```python
from build123d import *

# Parameters (mm, degrees)
TORUS001_R   = 3.1
BOX_W        = 135
BOX_H        = 90
BOX_DEPTH    = 75
POCKET_DEPTH = 70


with BuildPart() as torus001:
    # Torus001 → Torus001 (revolve)
    with BuildSketch(Plane(origin=(-20, 0, 79), x_dir=(1, 0, 0), z_dir=(0, -1, 0))):
        with Locations((35, 0)):
            Circle(TORUS001_R)
    revolve(axis=Axis((-20, 0, 79), (0, 0, 1)))


with BuildPart() as pocket:
    # Box → Box (new body)
    with BuildSketch(Plane.XY):
        with Locations((67.5, 45)):
            Rectangle(BOX_W, BOX_H)
    extrude(amount=BOX_DEPTH)

    # Cut001: cut Torus001
    add(torus001.part, mode=Mode.SUBTRACT)


with BuildPart() as pocket_1:
    # Cut001 placement: moved
    add(pocket.part.moved(Location((-65, -45, 3))))

    # Sketch → Pocket (cut)
    with BuildSketch(Plane(origin=(-65, -45, 3), x_dir=(1, 0, 0), z_dir=(0, 0, -1))):
        Polygon((20, 0), (20, -20), (0, -20), (0, -70), (20, -70), (20, -90), (110, -90), (110, -70), (135, -70), (135, -20), (110, -20), (110, 0), align=None)
    extrude(amount=-POCKET_DEPTH, mode=Mode.SUBTRACT)


solid = pocket_1.part
```
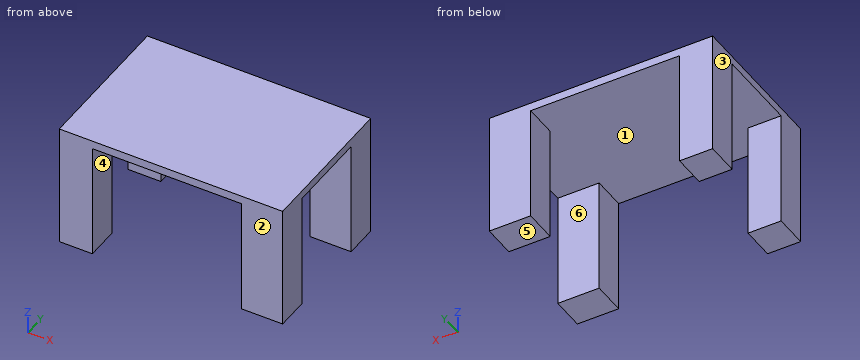
Input: part model. Units: mm. Frame: model coordinates. Face numbers are marked on the shaded views. A direction names the side the tool comes from. Give positions to 0.01 mm unless a question says otherwise; leave off trailing zeros. Order: outer loops, then holes, each group sorted by start corner. A loop starts at its lowest first (then second) coordinate and runs counter-clockwise, first axis right, second up. Notation, with made-up numbers: M 3.5,53 L 20.5,53 A10 ccw 20.5,61 Z; hole C 15.25,17.5 d9. An arc over 180 degrees is marked long. Return JSON: item names as keys, results as strings.
1) Section query C-C on y = 9. Output: boundary loops of the cut face in (x, z).
Taken from the geometry:
{"outline": "M -65,73 L 70,73 L 70,78 L -65,78 Z"}
2) Mould query, pull axis Y, two halves, no side actions, for the marked faces 1, 2 and 3. Classes: released by +Y, released by -Y, zero draft, split by the parting line, or undercut.
Taken from the geometry:
{"face 1": "undercut", "face 2": "released by -Y", "face 3": "zero draft"}
3) Contact query for flat-ended pins moving along their axis: pin 1 (4 mm diameter, centred on x = 17.5, y = 1.5, fed in from -Z); pin 2 (10 mm diameter, centred on y = -21.5, z = 25, fed in from -X). Output: stop coordinate, or through.
Taken from the geometry:
{"pin 1": "stops at z = 73", "pin 2": "stops at x = -65"}
4) Section query B-B on x = 59. Output: boundary loops of the cut face in (y, z), and give its area (3 significant figures).
Taken from the geometry:
{"outline": "M -45,3 L -25,3 L -25,73 L 25,73 L 25,3 L 45,3 L 45,78 L -45,78 Z", "area": "3,250 mm2"}
5) Section query A-A on z = 36. Output: boundary loops of the cut face in (x, y).
Taken from the geometry:
{"outline": "M -65,-45 L -45,-45 L -45,-25 L -65,-25 Z; M -65,25 L -45,25 L -45,45 L -65,45 Z; M 45,-45 L 70,-45 L 70,-25 L 45,-25 Z; M 45,25 L 70,25 L 70,45 L 45,45 Z"}
6) Line query: L1, parallel to X at y = 30, z = 37.5; L2, parallel to Z at x = 27.5, y = 28. Output: solid intervals per line, ascending. Write a range as [from, to].
Taken from the geometry:
{"L1": "x = [-65, -45], [45, 70]", "L2": "z = [73, 78]"}
7) Access query for the marked faces 4, 5 and 6. Directions: +Z, -Z, +X, -X, +Y, -Y. A direction counts if a zero-diameter tool reaches every point of the face in a straight line with its end or side. Return the directions, or none.
Taken from the geometry:
{"face 4": "-Z, +Y, -Y", "face 5": "-Z, +X, -X, +Y, -Y", "face 6": "-Z, +X, -X"}
8) Section query D-D on x = 36. Output: boundary loops of the cut face in (y, z), and give its area (3 significant figures).
Taken from the geometry:
{"outline": "M -45,73 L 45,73 L 45,78 L -45,78 Z", "area": "450 mm2"}
